```python
from build123d import *

# Parameters (mm, degrees)
F0_W     = 279.4
F0_H     = 203.2
F1_DEPTH = 6.35
F2_R     = 5.08
F3_R     = 5.08


with BuildPart() as f1:
    # F0 (on Top) → F1 (new body)
    with BuildSketch(Plane.XY):
        with Locations((139.7, -101.6)):
            Rectangle(F0_W, F0_H)
    extrude(amount=F1_DEPTH)

    # F2
    f2_edges = [f1.edges().sort_by_distance(p)[0] for p in [
        (139.7, -203.2, 0),
        (0, -101.6, 0),
    ]]
    fillet(f2_edges, radius=F2_R)

    # F3
    f3_edges = [f1.edges().sort_by_distance(p)[0] for p in [
        (279.4, -99.06, 0),
    ]]
    fillet(f3_edges, radius=F3_R)


solid = f1.part
```
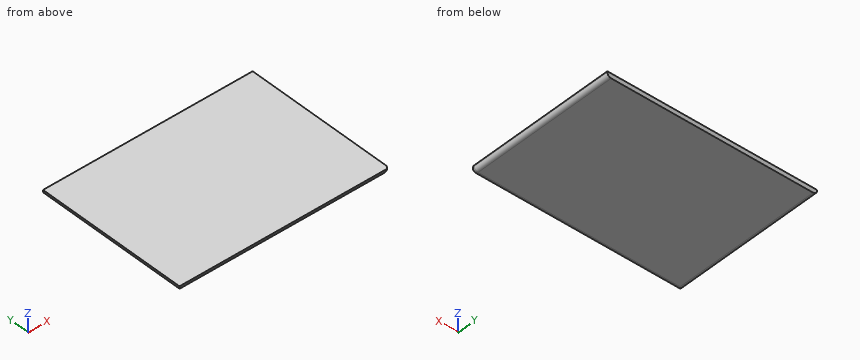
Geometry check sheet. Reference: the model listing, model coordinates, mm. Round coordinates to 2 decimals unless told otherwise and drop trailing zeros. Loops run counter-clockwise (first coordinate to the right, second up) from the corner with the lowest first, then second, coordinate; pieces in that order, holes last. Notation, with made-up numbers: M -38,37 L 4,37 A7 cw 4,47 Z; hole C -9,67.25 d5. An arc over 180 degrees is marked long. Return JSON: item names as keys, results as strings. Group by question number.
(1) Section check A-A, the plane z = 1.25. Enter the section's corners in (x, y), and give its area (3 significant figures).
(2) Go/stop test with flat-tipped pins: pin 1 (3 mm diameter, centred on y = -181.5, z = 3, fed in from -X); pin 2 (1 mm diameter, centred on x = 63.5, z = 2.5, fed in from -Y). Record where each tip stops, or that it passes through.
(3) Scan lines: line 1 along Y through (x, z) = (176, 4.25); line 2 along X through (y, z) = (-20, 4.25); line 3 along Y through (x, z) = (175, 4.5). Record each from-to range of solid material in increasing order. Write a range as [from, to].
Data:
{
 "1": {"outline": "M 1.74,-201.46 L 274.32,-201.46 A3.34 ccw 277.66,-198.12 L 277.66,0 L 1.74,0 Z", "area": "55,600 mm²"},
 "2": {"pin 1": "x = 0.03", "pin 2": "y = -202.75"},
 "3": {"line 1": "[-203.13, 0]", "line 2": "[0.07, 279.33]", "line 3": "[-203.17, 0]"}
}
